```python
from build123d import *

# Parameters (mm, degrees)
EXTRUDE_THIN1_DEPTH  = 15
SKETCH2_R            = 6.1
CUT_EXTRUDE1_DEPTH   = 62.306626885
FILLET1_R            = 12
FILLET1_OF_MIRROR1_R = 12
SKETCH3_W            = 30
SKETCH3_H            = 20
CUT_EXTRUDE2_DEPTH   = 63.472413912


with BuildPart() as part:
    # Sketch1 → Extrude-Thin1 (new, symmetric)
    with BuildSketch(Plane.XY):
        Polygon((-55, 4.5), (-28, 4.5), (-28, 9.5), (-25.5, 9.5), (-25.5, 16), (-22, 16), (-22, 21.5), (-16.5, 21.5), (-16.5, 27.05), (0, 27.05), (0, 30.05), (-19.5, 30.05), (-19.5, 24.5), (-25, 24.5), (-25, 19), (-28.5, 19), (-28.5, 12.5), (-31, 12.5), (-31, 7.5), (-55, 7.5), align=None)
    extrude_thin1 = extrude(amount=EXTRUDE_THIN1_DEPTH, both=True)

    # Sketch2 → Cut-Extrude1 (cut, through all)
    with BuildSketch(Plane(origin=(0, 7.5, 0), x_dir=(1, 0, 0), z_dir=(0, 1, 0))):
        with Locations(Location((-44, 0, 0), (0, 0, 270))):
            Circle(SKETCH2_R)
    cut_extrude1 = extrude(amount=-CUT_EXTRUDE1_DEPTH, mode=Mode.SUBTRACT)

    # Fillet1
    fillet1_edges = [part.edges().sort_by_distance(p)[0] for p in [
        (-55, 6, -15),
        (-55, 6, 15),
    ]]
    fillet(fillet1_edges, radius=FILLET1_R)

    # Mirror1: Extrude-Thin1, Cut-Extrude1 across plane
    add(extrude_thin1.mirror(Plane(origin=(0, 30.05, 15), x_dir=(0, 0, 1), z_dir=(1, 0, 0))))
    add(cut_extrude1.mirror(Plane(origin=(0, 30.05, 15), x_dir=(0, 0, 1), z_dir=(1, 0, 0))), mode=Mode.SUBTRACT)

    # Fillet1 of Mirror1
    fillet1_of_mirror1_edges = [part.edges().sort_by_distance(p)[0] for p in [
        (55, 6, -15),
        (55, 6, 15),
    ]]
    fillet(fillet1_of_mirror1_edges, radius=FILLET1_OF_MIRROR1_R)

    # Sketch3 → Cut-Extrude2 (cut, through all)
    with BuildSketch(Plane(origin=(0, 30.05, 0), x_dir=(1, 0, 0), z_dir=(0, 1, 0))):
        Rectangle(SKETCH3_W, SKETCH3_H)
    extrude(amount=-CUT_EXTRUDE2_DEPTH, mode=Mode.SUBTRACT)


solid = part.part
```
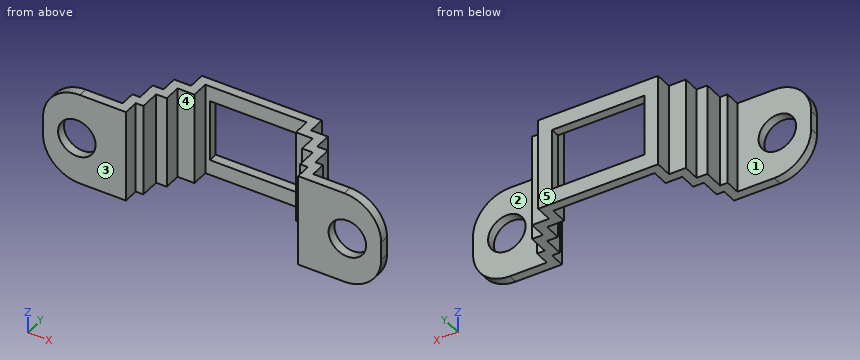
Work out the finished part from the listing and answer in its coordinate system (mm). Face numbers are marked on the shaded views. A direction names the side the tool comes from. Coordinates: 2 decimals unless noted, no trailing zeros. Write each loop counter-clockwise with the first axis right and the second up, starting at its lowest first coordinate (ties: lowest second). Pieces come first, ordered by that corner, then holes. Notation, with made-up numbers: (63, 62.5) - (78, 62.5) arc R26 cw to (78, 81.5) - close; hole circle Ø2 at (47.5, -17). An arc over 180 degrees is marked (long way). Answer as a JSON object with one key per item and string values.
Q1. Find section A-A (x = -13.5). Write down the section's boundary in (y, z), plus the area to 3 significant figures.
Results list:
{"outline": "(27.05, -15) - (30.05, -15) - (30.05, -10) - (27.05, -10) - close; (27.05, 10) - (30.05, 10) - (30.05, 15) - (27.05, 15) - close", "area": "30.0 mm^2"}
Q2. Find section C-C (z = 0). State how many separate pieces and enclosed holes the cut face has, plus the area to 3 significant figures.
Results list:
{"separate pieces": "4", "enclosed holes": "0", "area": "302 mm^2"}
Q3. Find section D-D (x = 27). Write down the section's boundary in (y, z).
Results list:
{"outline": "(9.5, -15) - (19, -15) - (19, 15) - (9.5, 15) - close"}
Q4. For a pull along X with two mould halves and no side action, classify the marked faces 4 and 5 as pulls with the +X half, pulls with the -X half, needs draft (parallel to the pull), parting line crosses it, or undercut.
Results list:
{"face 4": "undercut", "face 5": "needs draft"}
Q5. Given pin 1 Ø8 at (y, z) = (14.5, 11) entering from +X; pin 2 Ø1.2 at (x, z) = (26.5, -1) entering from -Y; pin 3 Ø1.5 at (y, z) = (28, -1.5) entering from +X; pin 4 Ø8 at (x, y) = (35, 15) entering from -Z, each flat-ended and moving along its own axis, determine where each tip first touches the part or whether it passes through.
Results list:
{"pin 1": "stops at x = 31", "pin 2": "stops at y = 9.5", "pin 3": "stops at x = 19.5", "pin 4": "passes through"}
Q6. Consider L1, parallel to X at y = 6.05, z = 0; L2, parallel to X at y = 8, z = 8; L3, parallel to X at y = 13, z = -2. Determine where each line is inside the solid, lowest interval first. Write a range as from..to.
Results list:
{"L1": "x = -55..-50.1, -37.9..-28, 28..37.9, 50.1..55", "L2": "x = -31..-28, 28..31", "L3": "x = -28.5..-25.5, 25.5..28.5"}
Q7. Find section B-B (y = 18). Write down the section's boundary in (x, z).
Results list:
{"outline": "(-28.5, -15) - (-22, -15) - (-22, 15) - (-28.5, 15) - close; (22, -15) - (28.5, -15) - (28.5, 15) - (22, 15) - close"}
Q8. Which of the six approach directions +Z, -Z, +X, -X, +Y, -Y give full straight-line access (tool end or side, diameter ignored) to the marked faces 1, 2 and 3?
Results list:
{"face 1": "+Z, -Z, -X, +Y", "face 2": "+Z, -Z, +X, +Y", "face 3": "+Z, -Z, +X, -X, -Y"}
